from build123d import *

# Parameters (mm, degrees)
F1_DEPTH      = 5
F3_DEPTH      = 5.001
F5_DEPTH      = 35
F6_W          = 5
F6_H          = 5
F7_DEPTH      = 90
F7_DEPTH_BACK = 90
F9_DEPTH      = 180.001
F10_T1_DEPTH  = 5
F10_T6_DEPTH  = 17.0072864353
F10_S7_R      = 12
F10_T8_DEPTH  = 11
F10_T9_DEPTH  = 30


# Not quite as in the source:
# - a fillet or chamfer that OpenCascade refuses, or shapes differently, is made with other operations: its cross-section is extruded or revolved along the edge and cut away or added


with BuildPart() as f1:
    # F0 (on Top) → F1 (new body)
    with BuildSketch(Plane.XY):
        Polygon((8.5036432176, -40), (-8.5036432176, -40), (-8.5036432176, -110), (0, -110), (8.5036432176, -110), align=None)
    extrude(amount=F1_DEPTH)

    # F2 (on face) → F3 (cut, through all)
    with BuildSketch(Plane.XY.offset(5)):
        with BuildLine():
            Line((-3.15, -67.75), (3.15, -67.75))
            Line((3.15, -67.75), (3.15, -63.4))
            ThreePointArc((3.15, -63.4), (0.75, -61), (3.15, -58.6))
            Line((3.15, -58.6), (3.15, -46.25))
            Line((3.15, -46.25), (-3.15, -46.25))
            Line((-3.15, -46.25), (-3.15, -50.6))
            ThreePointArc((-3.15, -50.6), (-0.75, -53), (-3.15, -55.4))
            Line((-3.15, -55.4), (-3.15, -67.75))
        make_face()
    extrude(amount=-F3_DEPTH, mode=Mode.SUBTRACT)

    # F4 (on face) → F5 (join)
    with BuildSketch(Plane.XZ.offset(110)):
        with BuildLine():
            ThreePointArc((8.5036432176, 5), (0, 8.5331202898), (-8.5036432176, 5))
            Line((-8.5036432176, 5), (8.5036432176, 5))
        make_face()
    extrude(amount=-F5_DEPTH)

    # F6 (on Right) → F7 (join, two sides)
    with BuildSketch(Plane.YZ) as f7_sk:
        with Locations((-42.5, 2.5)):
            Rectangle(F6_W, F6_H)
    extrude(amount=F7_DEPTH)
    extrude(f7_sk.sketch, amount=-F7_DEPTH_BACK)

    # F8 (on face) → F9 (cut, through all)
    with BuildSketch(Plane(origin=(-90, 0, 0), x_dir=(0, -1, 0), z_dir=(-1, 0, 0))):
        Polygon((40, 1), (42, 2), (42, 3), (40, 4), align=None)
    extrude(amount=-F9_DEPTH, mode=Mode.SUBTRACT)

    # F10: fillet of radius 5 on 5 edges, made by hand

    # F10_s2 → F10_t1 (join)
    with BuildSketch(Plane.XY):
        with BuildLine():
            ThreePointArc((-13.5036432176, -45), (-9.9681093117, -46.4644660941), (-8.5036432176, -50))
            Line((-8.5036432176, -50), (-8.5036432176, -45))
            Line((-8.5036432176, -45), (-13.5036432176, -45))
        make_face()
        with BuildLine():
            ThreePointArc((8.5036432176, -50), (9.9681093117, -46.4644660941), (13.5036432176, -45))
            Line((13.5036432176, -45), (8.5036432176, -45))
            Line((8.5036432176, -45), (8.5036432176, -50))
        make_face()
    extrude(amount=F10_T1_DEPTH)


with BuildPart() as f10_tool4:
    # F10_s5 → F10_t6 (new body)
    with BuildSketch(Plane.YZ.offset(-8.5036432176)):
        with BuildLine():
            ThreePointArc((-70, 5), (-73.5355339059, 6.4644660941), (-75, 10))
            Line((-75, 10), (-75, 5))
            Line((-75, 5), (-70, 5))
        make_face()
    extrude(amount=F10_T6_DEPTH)

    # F10_s7 → F10_t8 (intersect, symmetric)
    with BuildSketch(Plane.XZ.offset(72.5)):
        with Locations((0, -3.4668797102)):
            Circle(F10_S7_R)
    extrude(amount=F10_T8_DEPTH, both=True, mode=Mode.INTERSECT)


with BuildPart() as f1_1:
    add(f1.part)

    # F10_t3: union F10_tool4
    add(f10_tool4.part)

    # F10_s10 → F10_t9 (cut)
    with BuildSketch(Plane.XY.offset(-12.5)):
        with BuildLine():
            ThreePointArc((-8.5036432176, -105), (-7.0391771236, -108.5355339059), (-3.5036432176, -110))
            Line((-3.5036432176, -110), (-8.5036432176, -110))
            Line((-8.5036432176, -110), (-8.5036432176, -105))
        make_face()
        with BuildLine():
            ThreePointArc((8.5036432176, -105), (7.0391771236, -108.5355339059), (3.5036432176, -110))
            Line((3.5036432176, -110), (8.5036432176, -110))
            Line((8.5036432176, -110), (8.5036432176, -105))
        make_face()
    extrude(amount=F10_T9_DEPTH, mode=Mode.SUBTRACT)


solid = f1_1.part
Can you work these out from the model? Positions are in its coordinate system, mm. A direction names the side the tool comes from. Coordinates: 2 decimals unless noted, no trailing zeros. Order: outer loops, then holes, each group sorted by start corner. A loop starts at its lowest first (then second) coordinate and runs counter-clockwise, first axis right, second up. Notation, with made-up numbers: (49, -14.75) -> (62, -14.75) arc R32 ccw to (62, 23.25) -> close; hole circle Ø10 at (74, 27). An arc over 180 degrees is marked (long way). Use one line per item in the form item = value.
Q1. I need wall thicknesses on L1, parallel to X at y = -58.5, z = 2.5; L2, parallel to Y at x = 0, z = 2.25; L3, parallel to Y at x = -65, z = 0.75. Which ranges of each line are inside material? Lowest first, please.
From the geometry:
L1 = -8.5 to -3.15, 3.15 to 8.5
L2 = -110 to -67.75, -46.25 to -42
L3 = -45 to -40
Q2. Imagine slicing it at A-A, the plane y = -61. List the corners of the cut face in (x, z) for me, then the cut area to 3 significant figures.
From the geometry:
outline = (-8.5, 0) -> (-3.15, 0) -> (-3.15, 5) -> (-8.5, 5) -> close; (0.75, 0) -> (8.5, 0) -> (8.5, 5) -> (0.75, 5) -> close
area = 65.5 mm²
Q3. Which directions (+Z, -Z, +X, -X, +Y, -Y) give clear straight access to the entire face, cutting with the end or side of a thin tool? Please do faces 5 (the face through (0, -46.25, 3)), 6 (the face through (51, -45, 2)), 7 (the face through (-51, -45, 2)).
From the geometry:
face_5 = +Z, -Z
face_6 = +Z, -Z, +X, -Y
face_7 = +Z, -Z, -X, -Y
Q4. Will these pins go through, and if not, where does the flat tip stop? P1, Ø3.5, axis at y = -66, z = 2.5, coming from the -X side; P2, Ø2.5, axis at x = -55.5, z = 3, coming from the -Y side; P3, Ø1, axis at x = -15.5, z = 6.5, coming from the +Y side; P4, Ø0.8, axis at x = -12, z = 2.5, coming from the +Y side.
From the geometry:
P1 = -8.5
P2 = -45
P3 = through
P4 = -42
Q5. We'd pull the mould along X, two halves only. Please class faces 1 (the face through (-0.75, -52.95, 2.54)), 2 (the face through (9.929, -46.504, 2.465)), 3 (the face through (-0.12, -72.34, 5.58)), 4 (the face through (-8.504, -77, 2)): released by +X, released by -X, zero draft, split by the parting line, or undercut.
From the geometry:
face_1 = undercut
face_2 = released by +X
face_3 = zero draft
face_4 = released by -X
Q6. Imagine slicing it at C-C, the plane y = -81.5. List the corners of the cut face in (x, z) for me, then the cut area to 3 significant figures.
From the geometry:
outline = (-8.5, 0) -> (8.5, 0) -> (8.5, 5) arc R12 ccw to (-8.5, 5) -> close
area = 126 mm²
Q7. Imagine slicing it at B-B, the plane x = 52. List the corners of the cut face in (y, z) for me.
From the geometry:
outline = (-45, 0) -> (-40, 0) -> (-40, 1) -> (-42, 2) -> (-42, 3) -> (-40, 4) -> (-40, 5) -> (-45, 5) -> close
